```python
from build123d import *

# Parameters (mm, degrees)
SKETCH_W            = 95
SKETCH_H            = 160
PAD_DEPTH           = 1
SKETCH001_R         = 11.5
POCKET_DEPTH        = 1
SKETCH002_W         = 95
SKETCH002_H         = 160
PAD001_DEPTH        = 1
SKETCH003_R         = 6.5
PAD002_DEPTH        = 10
SKETCH004_R         = 6
POCKET001_DEPTH     = 9
SKETCH005_R         = 3
HOLE_DEPTH          = 25
HOLE001_D           = 3.4
HOLE001_DEPTH       = 25
HOLE001_CSINK_D     = 6
HOLE001_CSINK_ANGLE = 90
SKETCH007_W         = 2
SKETCH007_H         = 15
SKETCH007_W_2       = 15
SKETCH007_H_2       = 2
POCKET002_DEPTH     = 7


with BuildPart() as part:
    # Sketch → Pad (new body)
    with BuildSketch(Plane.XY):
        Rectangle(SKETCH_W, SKETCH_H)
    extrude(amount=PAD_DEPTH)

    # Sketch001 (on Face6 of Pad) → Pocket (cut)
    with BuildSketch(Plane.XY.offset(1)):
        with Locations((-32.5, 59)):
            Circle(SKETCH001_R)
        with Locations((-32.5, -1)):
            Circle(SKETCH001_R)
        with Locations((-32.5, -61)):
            Circle(SKETCH001_R)
        with Locations((33.5, 29)):
            Circle(SKETCH001_R)
        with Locations((33.5, -31)):
            Circle(SKETCH001_R)
    extrude(amount=-POCKET_DEPTH, mode=Mode.SUBTRACT)

    # Sketch002 (on Face5 of Pocket) → Pad001 (join)
    with BuildSketch(Plane.XY.offset(1)):
        Rectangle(SKETCH002_W, SKETCH002_H)
    extrude(amount=PAD001_DEPTH)

    # Sketch003 (on Face14 of Pad001) → Pad002 (join)
    with BuildSketch(Plane.XY.offset(2)):
        with Locations((-32.5, 59)):
            Circle(SKETCH003_R)
        with Locations((-32.5, -1)):
            Circle(SKETCH003_R)
        with Locations((33.5, 29)):
            Circle(SKETCH003_R)
        with Locations((33.5, -31)):
            Circle(SKETCH003_R)
        with Locations((-32.5, -61)):
            Circle(SKETCH003_R)
    extrude(amount=PAD002_DEPTH)

    # Sketch004 (on Face30 of Pad002) → Pocket001 (cut)
    with BuildSketch(Plane.XY.offset(12)):
        with Locations((-32.5, 59)):
            Circle(SKETCH004_R)
        with Locations((33.5, 29)):
            Circle(SKETCH004_R)
        with Locations((-32.5, -1)):
            Circle(SKETCH004_R)
        with Locations((33.5, -31)):
            Circle(SKETCH004_R)
        with Locations((-32.5, -61)):
            Circle(SKETCH004_R)
    extrude(amount=-POCKET001_DEPTH, mode=Mode.SUBTRACT)

    # Sketch005 (on Face40 of Pocket001) → Hole (cut)
    with BuildSketch(Plane.XY.offset(3)):
        with Locations((-32.5, 59)):
            Circle(SKETCH005_R)
        with Locations((33.5, 29)):
            Circle(SKETCH005_R)
        with Locations((-32.5, -1)):
            Circle(SKETCH005_R)
        with Locations((33.5, -31)):
            Circle(SKETCH005_R)
        with Locations((-32.5, -61)):
            Circle(SKETCH005_R)
    extrude(amount=-HOLE_DEPTH, mode=Mode.SUBTRACT)

    # Hole001
    with Locations(Plane(origin=(0, 0, 0), x_dir=(1, 0, 0), z_dir=(0, 0, -1))):
        with Locations((-42.5, 75), (42.5, 75), (-42.5, -75), (42.5, -75)):
            CounterSinkHole(HOLE001_D / 2, HOLE001_CSINK_D / 2, depth=HOLE001_DEPTH, counter_sink_angle=HOLE001_CSINK_ANGLE)

    # Sketch007 (on Face43 of Hole001) → Pocket002 (cut)
    with BuildSketch(Plane.XY.offset(12)):
        with Locations((-32.5, 59)):
            Rectangle(SKETCH007_W, SKETCH007_H)
        with Locations((-32.5, 59)):
            Rectangle(SKETCH007_W_2, SKETCH007_H_2)
        with Locations((32, 28.999954)):
            Rectangle(SKETCH007_W, SKETCH007_H)
        with Locations((32, 28.999655)):
            Rectangle(SKETCH007_W_2, SKETCH007_H_2)
        with Locations((-34, -1)):
            Rectangle(SKETCH007_W, SKETCH007_H)
        with Locations((-34, -1.000345)):
            Rectangle(SKETCH007_W_2, SKETCH007_H_2)
        with Locations((32, -31.000046)):
            Rectangle(SKETCH007_W, SKETCH007_H)
        with Locations((32, -30.999997)):
            Rectangle(SKETCH007_W_2, SKETCH007_H_2)
        with Locations((-34, -61.000017)):
            Rectangle(SKETCH007_W, SKETCH007_H)
        with Locations((-34, -61.000345)):
            Rectangle(SKETCH007_W_2, SKETCH007_H_2)
    extrude(amount=-POCKET002_DEPTH, mode=Mode.SUBTRACT)


solid = part.part
```
Could you check a few things on this model? Use its own coordinates, in mm. A direction names the side the tool comes from. Round coordinates to 2 decimals unless told otherwise and drop trailing zeros. Loops run counter-clockwise (first coordinate to the right, second up) from the corner with the lowest first, then second, coordinate; pieces in that order, holes last. Notation, with made-up numbers: (37.5, 78) - (96.5, 78) arc R15 ccw to (96.5, 84) - close; hole circle Ø1 at (-24.75, 6). An arc over 180 degrees is marked (long way). Answer in a Markdown table with one row per item. Add a question column.
(1) If we section it at C-C (z = 7.25): State how many separate pieces and enclosed holes the cut face has, plus the area to 3 significant figures.
(2) If we mould it in two halves opening along Y, with no side actions, what happens to faces 1 (the face through (-26.3, -59.05, 6.93)), 2 (the face through (-37.4, -4.9, 12))? For each: pulls with the +Y half, pulls with the -Y half, needs draft (parallel to the pull), parting line crosses it, or undercut.
(3) I need wall thicknesses on line 1 along Y through (x, z) = (-32.5, 0.5); line 2 along Y through (x, z) = (33.5, 10.25); line 3 along X through (y, z) = (-75, 1.6). Which ranges of each line are inside material? Lowest first, please.
(4) For faces 3 (the face through (22.01, 29.51, 0.51)), 4 (the face through (28.6, 25.1, 12)), 5 (the face through (39.7, -29.05, 6.93)), which set-ups out of +Z, -Z, +X, -X, +Y, -Y let a thin tool reach every point of the face, with its end or its side?
(5) If we section it at B-B (x = 42.5): Please give me the cut outline in (y, z).
(6) I'm going to push flat-ended pins straight in: pin 1 (6 mm diameter, centred on y = 22, z = 10, fed in from +X); pin 2 (7 mm diameter, centred on x = -29.5, y = -4.5, fed in from -Z); pin 3 (6 mm diameter, centred on x = -35, y = -59, fed in from +Z); pin 4 (0.6 mm diameter, centred on y = -1.5, z = 8, fed in from -X). Where does each tip first touch, or does it pass through?
(7) If we section it at D-D (y = 14): Please give me the cut outline in (x, z).
(8) If we section it at A-A (y = -75): Please give me the cut outline in (x, z), plus the area to 3 significant figures.
Model answer:
| question | item | result |
|---|---|---|
| 1 | separate pieces | 16 |
| 1 | enclosed holes | 0 |
| 1 | area | 81.6 mm² |
| 2 | face 1 | undercut |
| 2 | face 2 | needs draft |
| 3 | line 1 | y = -80 to -72.5, -49.5 to -12.5, 10.5 to 47.5, 70.5 to 80 |
| 3 | line 2 | y = -37.5 to -37, -25 to -24.5, 22.5 to 23, 35 to 35.5 |
| 3 | line 3 | x = -47.5 to -44.2, -40.8 to 40.8, 44.2 to 47.5 |
| 4 | face 3 | -Z |
| 4 | face 4 | +Z, +X, -X, +Y, -Y |
| 4 | face 5 | +Z |
| 5 | outline | (-80, 0) - (-78, 0) - (-76.7, 1.3) - (-76.7, 2) - (-80, 2) - close; (-73.3, 1.3) - (-72, 0) - (-38.16, 0) - (-38.16, 1) - (-23.84, 1) - (-23.84, 0) - (21.84, 0) - (21.84, 1) - (36.16, 1) - (36.16, 0) - (72, 0) - (73.3, 1.3) - (73.3, 2) - (-73.3, 2) - close; (76.7, 1.3) - (78, 0) - (80, 0) - (80, 2) - (76.7, 2) - close |
| 6 | pin 1 | stops at x = 38.62 |
| 6 | pin 2 | stops at z = 1 |
| 6 | pin 3 | stops at z = 12 |
| 6 | pin 4 | stops at x = -26.5 |
| 7 | outline | (-47.5, 0) - (47.5, 0) - (47.5, 2) - (-47.5, 2) - close |
| 8 | outline | (-47.5, 0) - (-45.5, 0) - (-44.2, 1.3) - (-44.2, 2) - (-47.5, 2) - close; (-40.8, 1.3) - (-39.5, 0) - (39.5, 0) - (40.8, 1.3) - (40.8, 2) - (-40.8, 2) - close; (44.2, 1.3) - (45.5, 0) - (47.5, 0) - (47.5, 2) - (44.2, 2) - close |
| 8 | area | 173 mm² |
